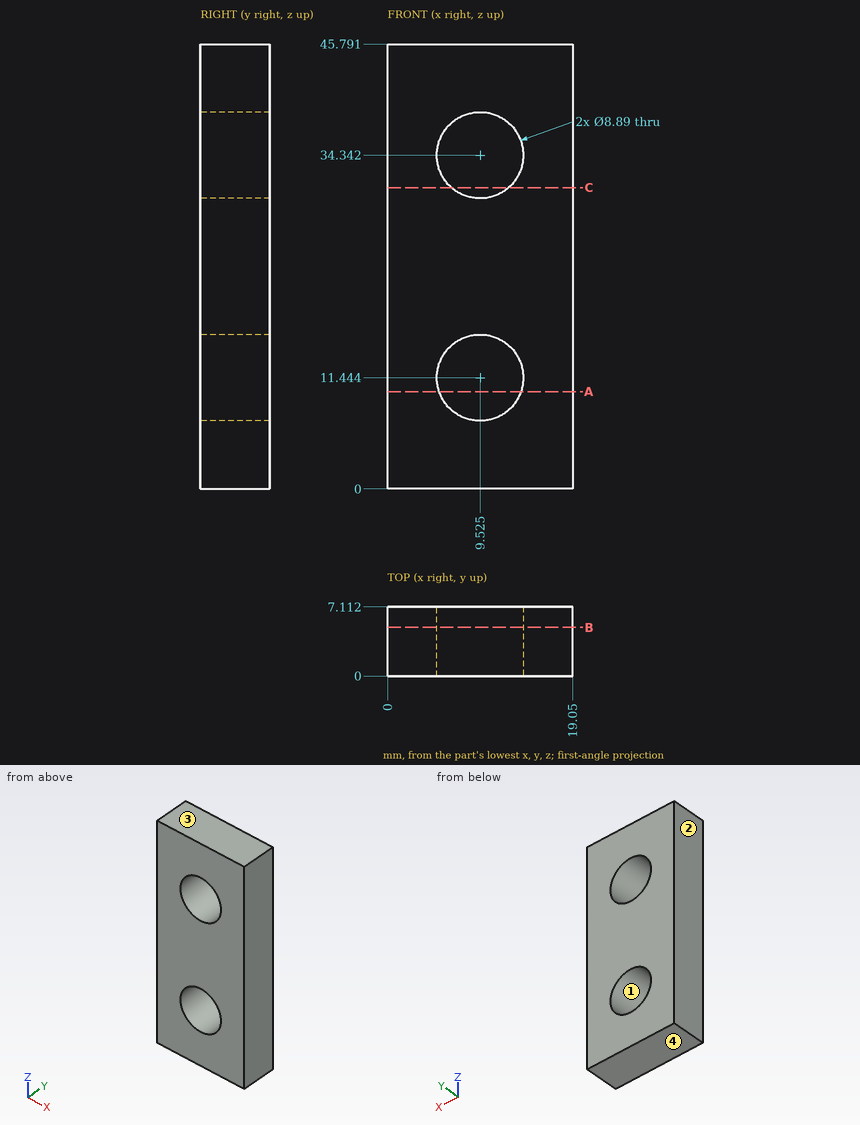
Here's the drawing with two shaded views (mm, measured from the low corner). I have some questions. Give positions to 0.01 mm unless a question says otherwise; leave off trailing zeros. Loops run counter-clockwise (first coordinate to the right, second up) from the corner with the lowest first, then second, coordinate; pieces in that order, holes last. Notation, with made-up numbers: M -12.75,86.25 L 27.25,86.25 A11 ccw 27.25,102.25 Z; hole C 59,12 d4. An arc over 180 degrees is marked long. One line per item, written item: value.
(1) Suppose I cut it at C-C on z = 31. List the corners of the cut face in (x, y) for me, plus the area to 3 significant figures.
Returned:
outline: M 0,0 L 6.59,0 L 6.59,7.11 L 0,7.11 Z; M 12.46,0 L 19.05,0 L 19.05,7.11 L 12.46,7.11 Z
area: 93.8 mm^2
(2) Suppose I cut it at B-B on y = 5. Count the separate pieces of the cut face and the enclosed holes in it, plus the area to 3 significant figures.
Returned:
separate pieces: 1
enclosed holes: 2
area: 748 mm^2
(3) We'd pull the mould along Z, two halves only. Please class the marked faces 1, 2, 3 and 4: released by +Z, released by -Z, zero draft, split by the parting line, or undercut.
Returned:
face 1: undercut
face 2: zero draft
face 3: released by +Z
face 4: released by -Z
(4) I need wall thicknesses on line 1 (Z direction, x = 9.5, y = 1.75); line 2 (Z direction, x = 10.75, y = 4.75) (1 decimal); line 3 (X direction, y = 4, z = 11.5). Which ranges of each line are inside material? Lowest first, please.
Returned:
line 1: 0 to 7, 15.89 to 29.9, 38.79 to 45.79
line 2: 0 to 7.2, 15.7 to 30.1, 38.6 to 45.8
line 3: 0 to 5.08, 13.97 to 19.05
(5) Suppose I cut it at A-A on z = 10. List the corners of the cut face in (x, y) for me, plus the area to 3 significant figures.
Returned:
outline: M 0,0 L 5.32,0 L 5.32,7.11 L 0,7.11 Z; M 13.73,0 L 19.05,0 L 19.05,7.11 L 13.73,7.11 Z
area: 75.7 mm^2
